Here's how the part is built. I have some questions about the finished solid (model axes, mm). Face numbers are marked on the shaded views. A direction names the side the tool comes from. Round coordinates to 2 decimals unless told otherwise and drop trailing zeros. Order: outer loops, then holes, each group sorted by start corner. A loop starts at its lowest first (then second) coordinate and runs counter-clockwise, first axis right, second up. Notation, with made-up numbers: (57.25, 68.5) -> (63.25, 68.5) arc R16 cw to (63.25, 94.5) -> close; hole circle Ø11 at (25, 17). An arc over 180 degrees is marked (long way). Answer in a Markdown table with one row per item.
```python
from build123d import *

# Parameters (mm, degrees)
F1_DEPTH = 90
F2_W     = 69
F2_H     = 2
F3_DEPTH = 75
F4_R     = 3.25
F5_DEPTH = 25
F6_SIZE  = 0.5


# Not quite as in the source:
# - a pattern or mirror of a feature is missing from the dataset's text; its kind, count and spacing are read off the source's solid


with BuildPart() as f1:
    # F0 (on Front) → F1 (new body, symmetric)
    with BuildSketch(Plane.XZ):
        with BuildLine():
            ThreePointArc((-1, 0), (-0.2928932188, -0.2928932188), (0, -1))
            Line((0, -1), (0, -250))
            Line((0, -250), (2, -250))
            Line((2, -250), (2, -1))
            ThreePointArc((2, -1), (1.1213203436, 1.1213203436), (-1, 2))
            Line((-1, 2), (-70, 2))
            Line((-70, 2), (-70, 0))
            Line((-70, 0), (-1, 0))
        make_face()
    extrude(amount=F1_DEPTH, both=True)

    # F2 (on face) → F3 (join)
    with BuildSketch(Plane.XZ.offset(90)):
        with Locations((-35.5, 1)):
            Rectangle(F2_W, F2_H)
    f3 = extrude(amount=F3_DEPTH)

    # F3_copies: F3 across plane
    add(f3.mirror(Plane.ZX))

    # F4 (on face) → F5 (cut)
    with BuildSketch(Plane.XY.offset(2)):
        with Locations((-60, 135)):
            Circle(F4_R)
        with Locations((-60, 0)):
            Circle(F4_R)
        with Locations((-60, -135)):
            Circle(F4_R)
    extrude(amount=-F5_DEPTH, mode=Mode.SUBTRACT)

    # F6
    f6_edges = [f1.edges().sort_by_distance(p)[0] for p in [
        (-63.25, 135, 2),
        (-56.75, 135, 1),
        (-63.25, 135, 0),
        (-63.25, 0, 2),
        (-56.75, 0, 1),
        (-63.25, 0, 0),
        (-63.25, -135, 2),
        (-56.75, -135, 1),
        (-63.25, -135, 0),
    ]]
    chamfer(f6_edges, length=F6_SIZE)


solid = f1.part
```
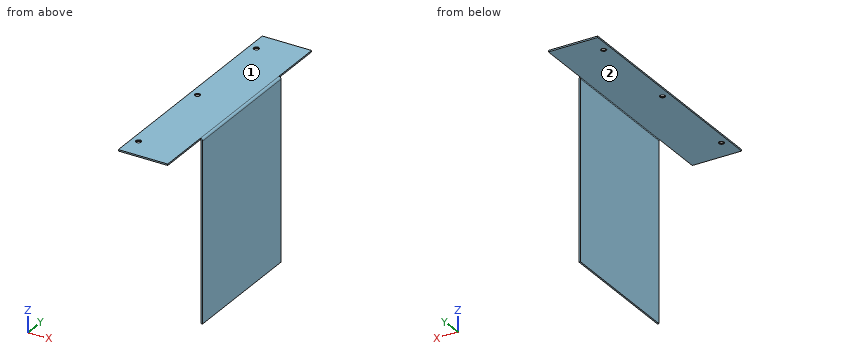
1. For pin 1 Ø1 at (x, y) = (-50.5, -28.5) entering from -Z; pin 2 Ø0.6 at (y, z) = (-138.5, 1.5) entering from +X; pin 3 Ø0.9 at (x, z) = (1, -186.5) entering from +Y, each with a flat end and sliding along its axis, tell me the tip position at first contact or that it passes through.
Numbers:
| item | result |
|---|---|
| pin 1 | stops at z = 0 |
| pin 2 | stops at x = -1 |
| pin 3 | stops at y = 90 |
2. Suppose I cut it at A-A on y = 121. Write out the boundary of the cut face in (x, z), then the cut area to 3 significant figures.
Numbers:
| item | result |
|---|---|
| outline | (-70, 0) -> (-1, 0) -> (-1, 2) -> (-70, 2) -> close |
| area | 138 mm2 |
3. Please list where these lines run through material, in increasing order: line 1 along Y through (x, z) = (-60, 1); line 2 along X through (y, z) = (-135, 1.2); line 3 along Z through (x, y) = (-61, 11.5).
Numbers:
| item | result |
|---|---|
| line 1 | y = -165 to -138.25, -131.75 to -3.25, 3.25 to 131.75, 138.25 to 165 |
| line 2 | x = -70 to -63.25, -56.75 to -1 |
| line 3 | z = 0 to 2 |
4. For the marked faces 1 and 2, which set-ups out of +Z, -Z, +X, -X, +Y, -Y let a thin tool reach every point of the face, with its end or its side?
Numbers:
| item | result |
|---|---|
| face 1 | +Z, +X, -X, +Y, -Y |
| face 2 | -Z, -X, +Y, -Y |
5. Suppose I cut it at B-B on z = -195. Write out the boundary of the cut face in (x, y), then the cut area to 3 significant figures.
Numbers:
| item | result |
|---|---|
| outline | (0, -90) -> (2, -90) -> (2, 90) -> (0, 90) -> close |
| area | 360 mm2 |
